Can you work these out from the drawing? Everything is in mm from the part's minimum corner. A direction names the side the tool comes from. Round coordinates to 2 decimals unless told otherwise and drop trailing zeros. Loops run counter-clockwise (first coordinate to the right, second up) from the corner with the lowest first, then second, coordinate; pieces in that order, holes last. Notation, with made-up numbers: (66, 27) -> (86, 27) arc R29 ccw to (86, 58) -> close; hole circle Ø1 at (-3, -15.75). An arc over 180 degrees is marked (long way). One line per item, written item: value.
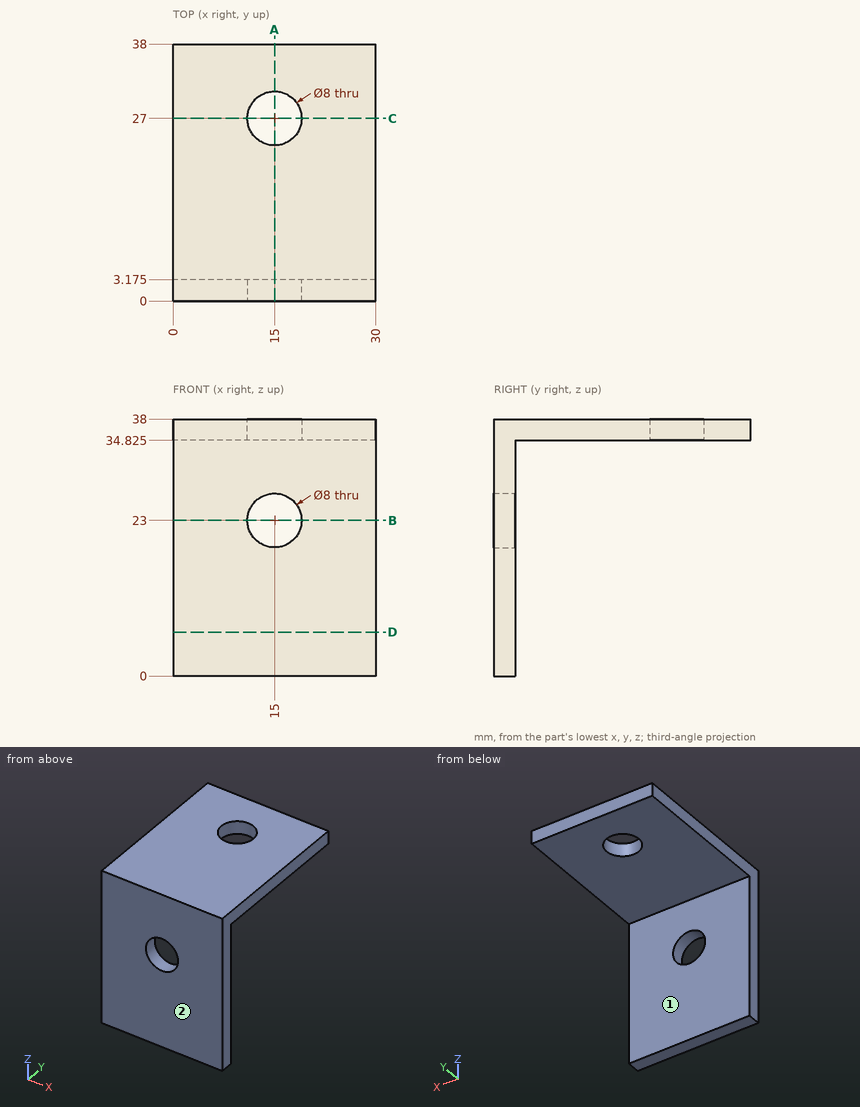
(1) Imagine slicing it at B-B on z = 23. Write out the boundary of the cut face in (x, y) (3 decimals), then the cut area to 4 significant figures.
Results below:
outline: (0, 0) -> (11, 0) -> (11, 3.175) -> (0, 3.175) -> close; (19, 0) -> (30, 0) -> (30, 3.175) -> (19, 3.175) -> close
area: 69.85 mm²
(2) For pin 1 Ø5 at (y, z) = (6, 31) entering from +X; pin 2 Ø15 at (x, y) = (15.5, 23.5) entering from -Z (3 decimals); pin 3 Ø9 at (x, z) = (13, 19) entering from +Y (3 decimals), each with a flat end and sliding along its axis, tell me the tip position at first contact or that it passes through.
Results below:
pin 1: passes through
pin 2: stops at z = 34.825
pin 3: stops at y = 3.175
(3) On a 3-axis mill with a long thin cutter (end or side, diameter ignored), from which of +Z, -Z, +X, -X, +Y, -Y can I reach the whole of each face in a straight line? I mean the marked faces 1 and 2. Say none if no direction works.
Results below:
face 1: -Z, +X, -X, +Y
face 2: +Z, -Z, +X, -X, -Y
(4) Please list where these lines run through material, in increasing order: L1, parallel to Y at x = 15, z = 36.45; L2, parallel to Y at x = 5.5, z = 34 (3 decimals); L3, parallel to Z at x = 15, y = 0.65.
Results below:
L1: y = 0 to 23, 31 to 38
L2: y = 0 to 3.175
L3: z = 0 to 19, 27 to 38
(5) Imagine slicing it at C-C on y = 27. Write out the boundary of the cut face in (x, z) (3 decimals), then the cut area to 4 significant figures.
Results below:
outline: (0, 34.825) -> (11, 34.825) -> (11, 38) -> (0, 38) -> close; (19, 34.825) -> (30, 34.825) -> (30, 38) -> (19, 38) -> close
area: 69.85 mm²
(6) Imagine slicing it at A-A on x = 15. Write out the boundary of the cut face in (y, z) (3 decimals), then the cut area to 3 significant figures.
Results below:
outline: (0, 0) -> (3.175, 0) -> (3.175, 19) -> (0, 19) -> close; (0, 27) -> (3.175, 27) -> (3.175, 34.825) -> (23, 34.825) -> (23, 38) -> (0, 38) -> close; (31, 34.825) -> (38, 34.825) -> (38, 38) -> (31, 38) -> close
area: 180 mm²
(7) Imagine slicing it at D-D on z = 6.5. Write out the boundary of the cut face in (x, y) (3 decimals).
Results below:
outline: (0, 0) -> (30, 0) -> (30, 3.175) -> (0, 3.175) -> close
